Read the model definition and answer for the solid it produces. Units are mm, in the model's axes. A direction names the side the tool comes from. Give positions to 0.01 mm unless a question says otherwise; leave off trailing zeros. Order: outer loops, then holes, each group sorted by start corner. A loop starts at its lowest first (then second) coordinate and runs counter-clockwise, first axis right, second up.
Item 1: The mould has two halves that part along X. Classify faces 1 (the face through (14.79, 27.676, 137.002)), 2 (the face through (27.324, 11.457, 772.998)), 3 (the face through (0, 27, 394)): +X half, -X half, draft (parallel to the pull), parting line (faces both ways), or undercut.
Item 2: A cutting plane is placed at A-A (z = 227.5). Write down the section's boundary in (x, y).
Item 3: Given pin 1 Ø6 at (y, z) = (31.5, 158) entering from -X; pin 2 Ø3 at (x, z) = (33, 163.5) entering from -Y, each flat-ended and moving along its own axis, determine where each tip first touches the part or whether it passes through.
Item 4: Which of the six approach directions +Z, -Z, +X, -X, +Y, -Y give full straight-line access (tool end or side, diameter ignored) to faces 4 (the face through (10, 19.5, 750)), 5 (the face through (27, 0, 394)), 6 (the face through (35.5, 15, 750))?
Item 5: Find the intervals of material crossed by line 1 along Z through (x, y) = (29, 5.5); line 2 along Z through (x, y) = (33, 5); line 3 along Y through (x, z) = (28, 732), in increasing order.
from build123d import *

# Parameters (mm, degrees)
ESQUISSE1_W             = 55
ESQUISSE1_H             = 55
BOSS_EXTRU_1_DEPTH      = 800
ENL_V_MAT_EXTRU_1_DEPTH = 30
ENL_V_START             = -55
ENL_V_MAT_EXTRU_3_DEPTH = 30
CHANFREIN1_SIZE         = 5


with BuildPart() as part:
    # Esquisse1 → Boss.-Extru.1 (new body)
    with BuildSketch(Plane.XY):
        with Locations((27.5, 27.5)):
            Rectangle(ESQUISSE1_W, ESQUISSE1_H)
    extrude(amount=BOSS_EXTRU_1_DEPTH)

    # Esquisse2 → Enlèv. mat.-Extru.1 (cut)
    with BuildSketch(Plane.XZ):
        with BuildLine():
            Line((35.5, 175), (35.5, 145))
            ThreePointArc((35.5, 145), (27.5, 137), (19.5, 145))
            Line((19.5, 145), (19.5, 175))
            ThreePointArc((19.5, 175), (27.5, 183), (35.5, 175))
        make_face()
        with BuildLine():
            Line((19.5, 735), (19.5, 765))
            ThreePointArc((19.5, 765), (27.5, 773), (35.5, 765))
            Line((35.5, 765), (35.5, 735))
            ThreePointArc((35.5, 735), (27.5, 727), (19.5, 735))
        make_face()
    extrude(amount=-ENL_V_MAT_EXTRU_1_DEPTH, mode=Mode.SUBTRACT)

    # Esquisse3<2> → Enlèv. mat.-Extru.3 (cut)
    with BuildSketch(Plane(origin=(55, 0, 0), x_dir=(0, 0, -1), z_dir=(1, 0, 0)).offset(ENL_V_START)):
        with BuildLine():
            Line((-175, 35.5), (-145, 35.5))
            ThreePointArc((-145, 35.5), (-137, 27.5), (-145, 19.5))
            Line((-145, 19.5), (-175, 19.5))
            ThreePointArc((-175, 19.5), (-183, 27.5), (-175, 35.5))
        make_face()
        with BuildLine():
            Line((-765, 35.5), (-735, 35.5))
            ThreePointArc((-735, 35.5), (-727, 27.5), (-735, 19.5))
            Line((-735, 19.5), (-765, 19.5))
            ThreePointArc((-765, 19.5), (-773, 27.5), (-765, 35.5))
        make_face()
    extrude(amount=ENL_V_MAT_EXTRU_3_DEPTH, mode=Mode.SUBTRACT)

    # Chanfrein1
    chanfrein1_edges = [part.edges().sort_by_distance(p)[0] for p in [
        (0, 55, 400),
        (55, 55, 400),
        (55, 0, 400),
        (0, 0, 400),
    ]]
    chamfer(chanfrein1_edges, length=CHANFREIN1_SIZE)


solid = part.part
Response values:
1. face 1: draft
1. face 2: undercut
1. face 3: -X half
2. outline: (0, 5) - (5, 0) - (50, 0) - (55, 5) - (55, 50) - (50, 55) - (5, 55) - (0, 50) - close
3. pin 1: stops at x = 30
3. pin 2: stops at y = 30
4. face 4: -X
4. face 5: +Z, -Z, +X, -X, -Y
4. face 6: -Y
5. line 1: z = 0 to 137.14, 182.86 to 727.14, 772.86 to 800
5. line 2: z = 0 to 139.19, 180.81 to 729.19, 770.81 to 800
5. line 3: y = 34.92 to 55
